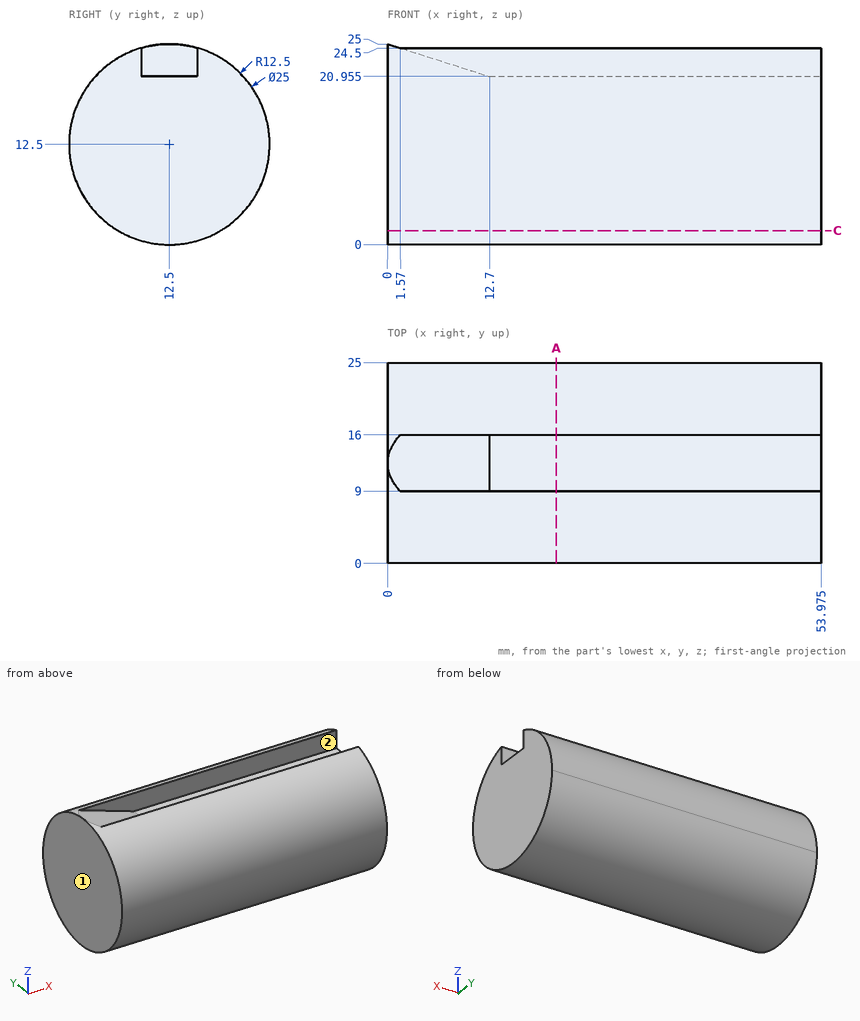
Input: dimensioned drawing with shaded views. Units: mm. Origin: part minimum x, y, z. Give positions to 0.01 mm unless a question says otherwise; leave off trailing zeros. Write each loop counter-clockwise with the first axis right and the second up, starting at its lowest first coordinate (ties: lowest second). Pieces come first, ordered by that corner, then holes. Notation, with made-up numbers: M 74,-27 L 113,-27 A15 ccw 113,-1 Z; hole C 39,69 d4. An arc over 180 degrees is marked long. Return JSON: item names as keys, results as strings. Group by question number.
1) Cut plane C-C, the plane z = 1.75. Output: boundary loops of the cut face in (x, y) (1 decimal).
2) Material intervals for line 1 along Y through (x, z) = (52, 12.25); line 2 along Y through (x, z) = (50, 23.5); line 3 along Y through (x, z) = (15.5, 13.75), sorted ascending. Write a range as [from, to].
3) Pin query (flat end, axial travel): P1, Ø6, axis at x = 44, z = 4, coming from the -Y side (3 decimals); P2, Ø1.5, axis at x = 10, y = 7.5, coming from the +Z side (1 decimal); P3, Ø10, axis at x = 18, z = 18.5, coming from the +Y side. Return the tip coordinate at first contact, or that it passes through.
4) Cut plane A-A, the plane x = 21. Output: boundary loops of the cut face in (y, z) (3 decimals), plus the area to 3 significant figures.
5) Pull-direction query (Y, two-part tool) for the marked faces 1 and 2; classes: pulls with the +Y half, pulls with the -Y half, needs draft (parallel to the pull), parting line crosses it, or undercut.
Recorded:
{
 "1": {"outline": "M 0,6.1 L 54,6.1 L 54,18.9 L 0,18.9 Z"},
 "2": {"line 1": "y = [0, 25]", "line 2": "y = [6.56, 9], [16, 18.44]", "line 3": "y = [0.06, 24.94]"},
 "3": {"P1": "stops at y = 1.275", "P2": "stops at z = 24.3", "P3": "stops at y = 24.96"},
 "4": {"outline": "M 9,20.955 L 9,24.5 A12.5 ccw long 16,24.5 L 16,20.955 Z", "area": "464 mm²"},
 "5": {"face 1": "needs draft", "face 2": "undercut"}
}
